For this review, take the finished solid that the model builds, in its own axes (mm). Give positions to 0.01 mm unless a question says otherwise; leave off trailing zeros. Loops run counter-clockwise (first coordinate to the right, second up) from the corner with the lowest first, then second, coordinate; pieces in that order, holes last. Notation, with made-up numbers: (40, -12.75) - (70, -12.75) arc R15 ccw to (70, 9.25) - close; hole circle Ø9 at (88, 0.25). An arc over 180 degrees is marked (long way). Answer in a Markdown table with one row per item.
```python
from build123d import *

# Parameters (mm, degrees)
F0_R     = 7.5
F0_R_2   = 5.25
F0_R_3   = 38.5
F1_DEPTH = 11.5
F2_SIZE2 = 1
F2_SIZE  = 1
F3_SIZE2 = 3
F3_SIZE  = 3
F4_SIZE2 = 1
F4_SIZE  = 1


with BuildPart() as f1:
    # F0 (on Front) → F1 (new body)
    with BuildSketch(Plane.XZ):
        with BuildLine():
            ThreePointArc((6.99611, 104.766667), (0, 98), (-6.99611, 104.766667))
            ThreePointArc((-6.99611, 104.766667), (-105, 0), (-6.99611, -104.766667))
            ThreePointArc((-6.99611, -104.766667), (0, -98), (6.99611, -104.766667))
            ThreePointArc((6.99611, -104.766667), (105, 0), (6.99611, 104.766667))
        make_face()
        with Locations((-59.534948, -60.667866)):
            Circle(F0_R, mode=Mode.SUBTRACT)
        with Locations((-82.307387, -21.224844)):
            Circle(F0_R, mode=Mode.SUBTRACT)
        with Locations((-45.899346, -26.5)):
            Circle(F0_R_2, mode=Mode.SUBTRACT)
        with Locations((0, -53)):
            Circle(F0_R_2, mode=Mode.SUBTRACT)
        with Locations((59.534948, -60.667866)):
            Circle(F0_R, mode=Mode.SUBTRACT)
        with Locations((45.899346, -26.5)):
            Circle(F0_R_2, mode=Mode.SUBTRACT)
        with Locations((82.307387, -21.224844)):
            Circle(F0_R, mode=Mode.SUBTRACT)
        with Locations((-45.899346, 26.5)):
            Circle(F0_R_2, mode=Mode.SUBTRACT)
        with Locations((-22.772439, 81.89271)):
            Circle(F0_R, mode=Mode.SUBTRACT)
        Circle(F0_R_3, mode=Mode.SUBTRACT)
        with Locations((45.899346, 26.5)):
            Circle(F0_R_2, mode=Mode.SUBTRACT)
        with Locations((0, 53)):
            Circle(F0_R_2, mode=Mode.SUBTRACT)
        with Locations((22.772439, 81.89271)):
            Circle(F0_R, mode=Mode.SUBTRACT)
    extrude(amount=F1_DEPTH)

    # F2
    f2_edges = [f1.edges().sort_by_distance(p)[0] for p in [
        (0, -11.5, 98),
        (105, -11.5, 0),
        (-105, -11.5, 0),
        (-30.272439, -11.5, 81.89271),
        (15.272439, -11.5, 81.89271),
        (-5.25, -11.5, 53),
        (40.649346, -11.5, 26.5),
        (40.649346, -11.5, -26.5),
        (74.807387, -11.5, -21.224844),
        (52.034948, -11.5, -60.667866),
        (-5.25, -11.5, -53),
        (-67.034948, -11.5, -60.667866),
        (-89.807387, -11.5, -21.224844),
        (-51.149346, -11.5, -26.5),
        (-51.149346, -11.5, 26.5),
        (0, -11.5, -98),
    ]]
    chamfer(f2_edges, length=F2_SIZE, length2=F2_SIZE2)

    # F3
    f3_edges = [f1.edges().sort_by_distance(p)[0] for p in [
        (-38.5, -11.5, 0),
    ]]
    chamfer(f3_edges, length=F3_SIZE, length2=F3_SIZE2)

    # F4
    f4_edges = [f1.edges().sort_by_distance(p)[0] for p in [
        (105, 0, 0),
        (-105, 0, 0),
        (0, 0, 98),
        (15.272439, 0, 81.89271),
        (-30.272439, 0, 81.89271),
        (-51.149346, 0, 26.5),
        (74.807387, 0, -21.224844),
        (40.649346, 0, 26.5),
        (40.649346, 0, -26.5),
        (-5.25, 0, -53),
        (-51.149346, 0, -26.5),
        (-89.807387, 0, -21.224844),
        (0, 0, -98),
        (-67.034948, 0, -60.667866),
        (52.034948, 0, -60.667866),
        (-5.25, 0, 53),
        (-38.5, 0, 0),
    ]]
    chamfer(f4_edges, length=F4_SIZE, length2=F4_SIZE2)


solid = f1.part
```
1. Clearance check with flat-ended pins moving along their axes: pin 1 (8.5 mm diameter, centred on x = -45.9, z = -26.5, fed in from +Y); pin 2 (24 mm diameter, centred on x = 82.31, z = -21.22, fed in from -Y); pin 3 (1.5 mm diameter, centred on x = -52, y = -7, fed in from +Z); pin 4 (2 mm diameter, centred on x = -54, y = -4, fed in from -Z). State where each tip first meets the part, or that it passes through.
Values:
| item | result |
|---|---|
| pin 1 | passes through |
| pin 2 | stops at y = -11.5 |
| pin 3 | stops at z = 91.64 |
| pin 4 | stops at z = -90.64 |
2. Mouldability with a two-part tool opening along X and no side actions: class faces 1 (the face through (104.977, -5.684, -2.211)), 2 (the face through (-51.144, -5.684, -26.269)) as released by +X, released by -X, zero draft, split by the parting line, or undercut.
Values:
| item | result |
|---|---|
| face 1 | released by +X |
| face 2 | undercut |
3. Wall thickness on line 1 (Z direction, x = 0, y = -6.75); line 2 (Z direction, x = -19.5, y = -4.75); line 3 (X direction, y = -1.5, z = 31): over which ranges is each line inside the solid? List them lowest first. Write a range as [from, to].
Values:
| item | result |
|---|---|
| line 1 | z = [-98, -58.25], [-47.75, -38.5], [38.5, 47.75], [58.25, 98] |
| line 2 | z = [-103.17, -33.2], [33.2, 75.14], [88.64, 103.17] |
| line 3 | x = [-100.32, -48.6], [-43.2, -22.83], [22.83, 43.2], [48.6, 100.32] |
4. We need section B-B, the plane z = 0. Give the boundary of the cut face in (x, y), and give its area (3 significant figures).
Values:
| item | result |
|---|---|
| outline | (-105, -10.5) - (-104, -11.5) - (-41.5, -11.5) - (-38.5, -8.5) - (-38.5, -1) - (-39.5, 0) - (-104, 0) - (-105, -1) - close; (38.5, -8.5) - (41.5, -11.5) - (104, -11.5) - (105, -10.5) - (105, -1) - (104, 0) - (39.5, 0) - (38.5, -1) - close |
| area | 1,520 mm^2 |
5. We need section A-A, the plane x = 0. Count the separate pieces of the cut face and the enclosed holes in it, and give its area (3 significant figures).
Values:
| item | result |
|---|---|
| separate pieces | 4 |
| enclosed holes | 0 |
| area | 1,110 mm^2 |
